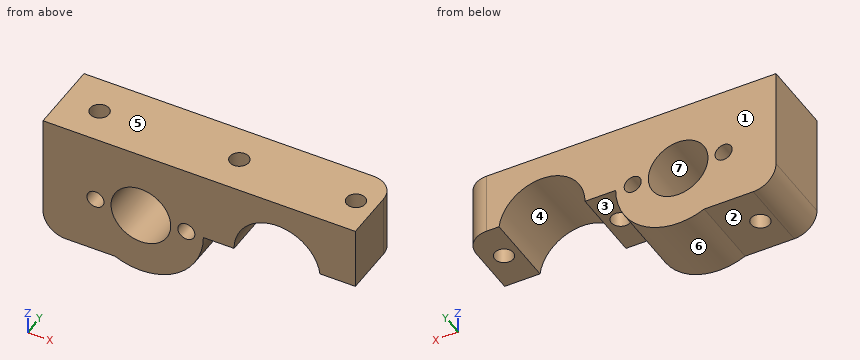
```python
from build123d import *

# Parameters (mm, degrees)
SKETCH1_R               = 5.25
SKETCH1_R_2             = 1.5
BOSS_EXTRUDE4_DEPTH     = 13
FILLET2_R               = 4
CUT_EXTRUDE1_DEPTH      = 40.402671632
CUT_EXTRUDE1_DEPTH_BACK = 40.402671632
SKETCH2_R               = 1.65
FILLET3_R               = 4


with BuildPart() as part:
    # Sketch1 → Boss-Extrude4 (new body)
    with BuildSketch(Plane(origin=(0, 0, 0), x_dir=(1, 0, 0), z_dir=(0, 1, 0))):
        with BuildLine():
            Line((-16.582575695, 10), (-29.23303836, 10))
            Line((-29.23303836, 10), (-29.23303836, -12))
            Line((-29.23303836, -12), (25.76696164, -12))
            Line((25.76696164, -12), (25.76696164, -1))
            Line((25.76696164, -1), (19.533923281, -1))
            ThreePointArc((19.533923281, -1), (11.498909656, -7.583462828), (4.4, 0))
            Line((4.4, 0), (-1, 0))
            ThreePointArc((-1, 0), (-6.058970318, 9.257654472), (-16.582575695, 10))
        make_face()
        with Locations(Location((-12, 0, 0), (0, 0, 90))):
            Circle(SKETCH1_R, mode=Mode.SUBTRACT)
        with Locations(Location((-4, 0, 0), (0, 0, 90))):
            Circle(SKETCH1_R_2, mode=Mode.SUBTRACT)
        with Locations(Location((-20, 0, 0), (0, 0, 90))):
            Circle(SKETCH1_R_2, mode=Mode.SUBTRACT)
    extrude(amount=BOSS_EXTRUDE4_DEPTH)

    # Fillet2
    fillet2_edges = [part.edges().sort_by_distance(p)[0] for p in [
        (25.76696164, 13, 6.5),
    ]]
    fillet(fillet2_edges, radius=FILLET2_R)

    # Sketch2 → Cut-Extrude1 (cut, two sides: drawn at the far end of the back side and taken through both)
    with BuildSketch(Plane.XY.offset(12).offset(-CUT_EXTRUDE1_DEPTH_BACK)):
        with Locations((22.26696164, 6.5)):
            Circle(SKETCH2_R)
        with Locations((1.73303836, 6.5)):
            Circle(SKETCH2_R)
        with Locations(Location((-22.73303836, 6.238089535, 0), (0, 0, 180))):
            Circle(SKETCH2_R)
    extrude(amount=CUT_EXTRUDE1_DEPTH + CUT_EXTRUDE1_DEPTH_BACK, mode=Mode.SUBTRACT)

    # Fillet3
    fillet3_edges = [part.edges().sort_by_distance(p)[0] for p in [
        (-29.23303836, 6.5, -10),
    ]]
    fillet(fillet3_edges, radius=FILLET3_R)


solid = part.part
```
CAD build for the part. Positions are in the model's coordinates, mm. Face numbers are marked on the shaded views. A direction names the side the tool comes from. Round coordinates to 2 decimals unless told otherwise and drop trailing zeros. Loops run counter-clockwise (first coordinate to the right, second up) from the corner with the lowest first, then second, coordinate; pieces in that order, holes last. Notation, with made-up numbers: M -22,69 L -11,69 A17 cw -11,87 Z; hole C 56,-22.5 d6. An arc over 180 degrees is marked long. Use a Markdown table: item, result. Add a question column.
(1) Flat gauge pins, fed straight in: pin 1 (5 mm diameter, centred on x = 23.5, y = 7.5, fed in from -Z); pin 2 (5 mm diameter, centred on y = 8, z = -2, fed in from +X). Where does each tip first touch, or does it go through?
(2) Cut at D-D (x = -4). Give the cut face in (y, z), and give its area (3 significant figures).
(3) Pull direction X, two halves, no side cores. Call the marked faces 4, 5, 6 and 7: +X half, -X half, draft (parallel to the pull), parting line (faces both ways), or undercut.
(4) Drill centre lines: line 1 (X direction, y = 4.5, z = -1.25); line 2 (Z direction, x = -20, y = 6.75); line 3 (X direction, y = 11.25, z = 3.75). Where is each one in solid material? Low to high.
(5) Which spindle directions (+Z, -Z, +X, -X, +Y, -Y) get a long thin tool onto all of the face, cutting with end or side? Do the marked faces 1, 2 and 3. Say none if no direction does.
(6) Cut at C-C (z = 10.25). Give the cut face in (x, y).
(7) Cut at B-B (y = 1.25). Give the cut face in (x, z).
(8) Cut at A-A (x = -20). Give the cut face in (y, z), and give its area (3 significant figures).
Geometry says:
| question | item | result |
|---|---|---|
| 1 | pin 1 | stops at z = 1 |
| 1 | pin 2 | stops at x = 4.42 |
| 2 | outline | M 0,-7.55 L 13,-7.55 L 13,-1.5 L 0,-1.5 Z; M 0,1.5 L 13,1.5 L 13,12 L 0,12 Z |
| 2 | area | 215 mm² |
| 3 | face 4 | undercut |
| 3 | face 5 | draft |
| 3 | face 6 | parting line |
| 3 | face 7 | undercut |
| 4 | line 1 | x = -29.23 to -20.83, -19.17 to -17.1, -6.9 to -4.83, -3.17 to -1.07 |
| 4 | line 2 | z = -10 to -1.5, 1.5 to 12 |
| 4 | line 3 | x = -29.23 to -15.67, -8.33 to 5.39, 18.61 to 25.07 |
| 5 | face 1 | +Z, -Z, +X, -X, +Y |
| 5 | face 2 | -Z, -X, +Y, -Y |
| 5 | face 3 | -Z, +X, +Y, -Y |
| 6 | outline | M -29.23,0 L 25.77,0 L 25.77,9 A4 ccw 21.77,13 L -29.23,13 Z; hole C -22.73,6.24 d3.3; hole C 1.73,6.5 d3.3; hole C 22.27,6.5 d3.3 |
| 7 | outline | M -29.23,-6 A4 ccw -25.23,-10 L -16.58,-10 A11 ccw -1,0 L 4.4,0 A7.6 cw 19.53,1 L 25.77,1 L 25.77,12 L -29.23,12 Z; hole C -20,0 d3; hole C -12,0 d10.5; hole C -4,0 d3 |
| 8 | outline | M 0,-10 L 13,-10 L 13,-1.5 L 0,-1.5 Z; M 0,1.5 L 13,1.5 L 13,12 L 0,12 Z |
| 8 | area | 247 mm² |
